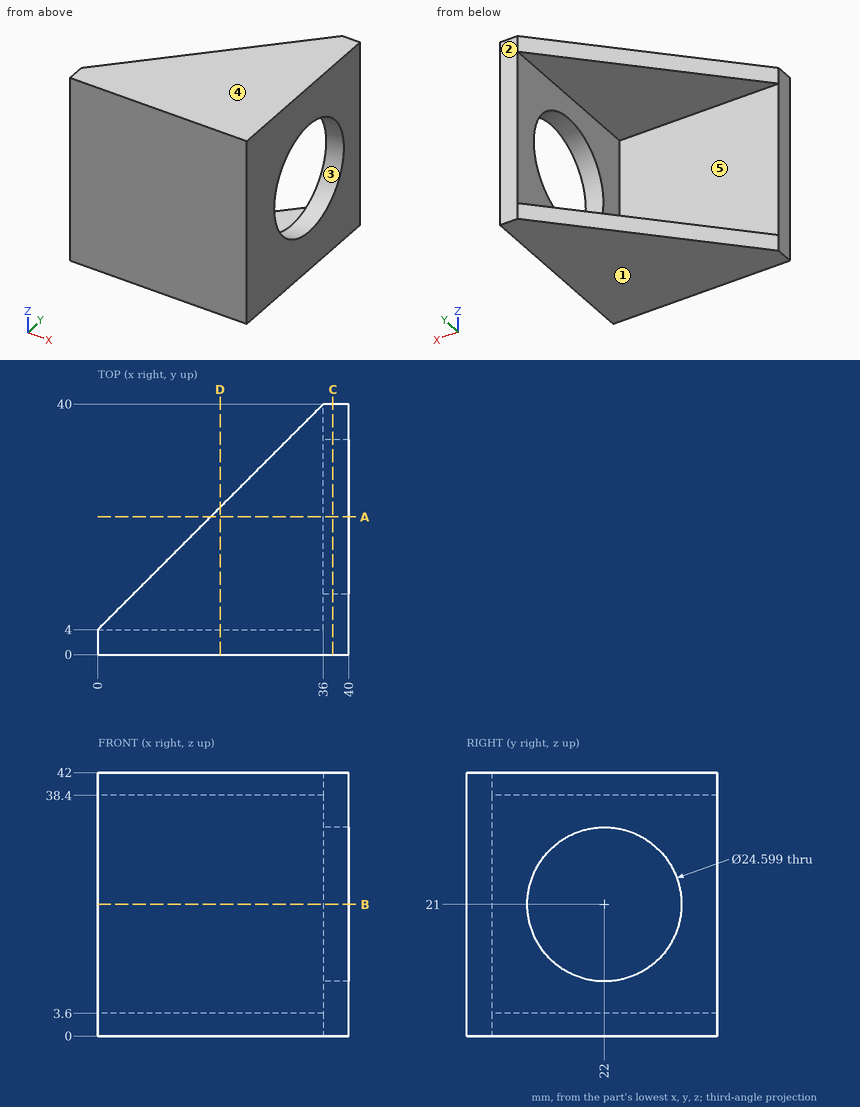
Design review of the part shown in the three views and the two pictorial views. Dimensions are in mm from the part's minimum x, y and z. A direction names the side the tool comes from. Round coordinates to 2 decimals unless told otherwise and drop trailing zeros. Loops run counter-clockwise (first coordinate to the right, second up) from the corner with the lowest first, then second, coordinate; pieces in that order, holes last. Notation, with made-up numbers: M 61.5,35.5 L 110.5,35.5 A16 cw 110.5,43.5 Z; hole C -38,44 d7. An arc over 180 degrees is marked long. Write item = value, one per line.
Item 1: Take a section at B-B on z = 21. Write out the cut boundary in (x, y), then the cut area to 3 significant figures.
Return value:
outline = M 0,0 L 40,0 L 40,9.7 L 36,9.7 L 36,4 L 0,4 Z; M 36,34.3 L 40,34.3 L 40,40 L 36,40 Z
area = 206 mm2
Item 2: Machinability: for the marked faces 4 and 5, which of the approach directions +Z, -Z, +X, -X, +Y, -Y give a long, thin tool a straight path to every point of the face, cutting with its end or side? Answer none if there is none.
Return value:
face_4 = +Z, +X, -X, +Y, -Y
face_5 = -X, +Y
Item 3: For line 1 (Z direction, x = 30, y = 25.5); line 2 (Z direction, x = 37, y = 22); line 3 (X direction, y = 19, z = 4.5), list the stretches that pass through material, from the lowest coordinate up. Write a range as [from, to].
Return value:
line_1 = [0, 3.6], [38.4, 42]
line_2 = [0, 8.7], [33.3, 42]
line_3 = [36, 40]
Item 4: Take a section at C-C on x = 37.5. Write out the cut boundary in (y, z).
Return value:
outline = M 0,0 L 40,0 L 40,42 L 0,42 Z; hole C 22,21 d24.6
Item 5: The part is to be moulded in two halves that separate along Y. For the marked faces 1, 2 and 3, say which applies: released by +Y, released by -Y, zero draft, split by the parting line, or undercut.
Return value:
face_1 = zero draft
face_2 = released by +Y
face_3 = undercut
Item 6: Take a section at A-A on y = 22. Write out the cut boundary in (x, z), then the cut area to 3 significant figures.
Return value:
outline = M 18,0 L 40,0 L 40,8.7 L 36,8.7 L 36,3.6 L 18,3.6 Z; M 18,38.4 L 36,38.4 L 36,33.3 L 40,33.3 L 40,42 L 18,42 Z
area = 199 mm2
Item 7: Take a section at D-D on x = 19.5. Write out the cut boundary in (y, z).
Return value:
outline = M 0,0 L 23.5,0 L 23.5,3.6 L 4,3.6 L 4,38.4 L 23.5,38.4 L 23.5,42 L 0,42 Z
Item 8: Insertion check: P1, Ø10.5, axis at y = 23.5, z = 17.5, coming from the -X side; P2, Ø6, axis at y = 11, z = 30, coming from the -X side; P3, Ø3, axis at x = 31.5, z = 7.5, coming from the -Y side; P4, Ø3, axis at x = 14.5, z = 32, coming from the +Y side. Each pin has a flat end and moves straight along its axis. Give the tip position at first contact, or say it passes through.
Return value:
P1 = through
P2 = 36
P3 = 0
P4 = 4
